The drawing under review shows one solid part. Ordinate dimensions are in mm from its lowest x, y, z. Coordinates: 2 decimals unless noted, no trailing zeros. Order: outer loops, then holes, each group sorted by start corner. A loop starts at its lowest first (then second) coordinate and runs counter-clockwise, first axis right, second up.
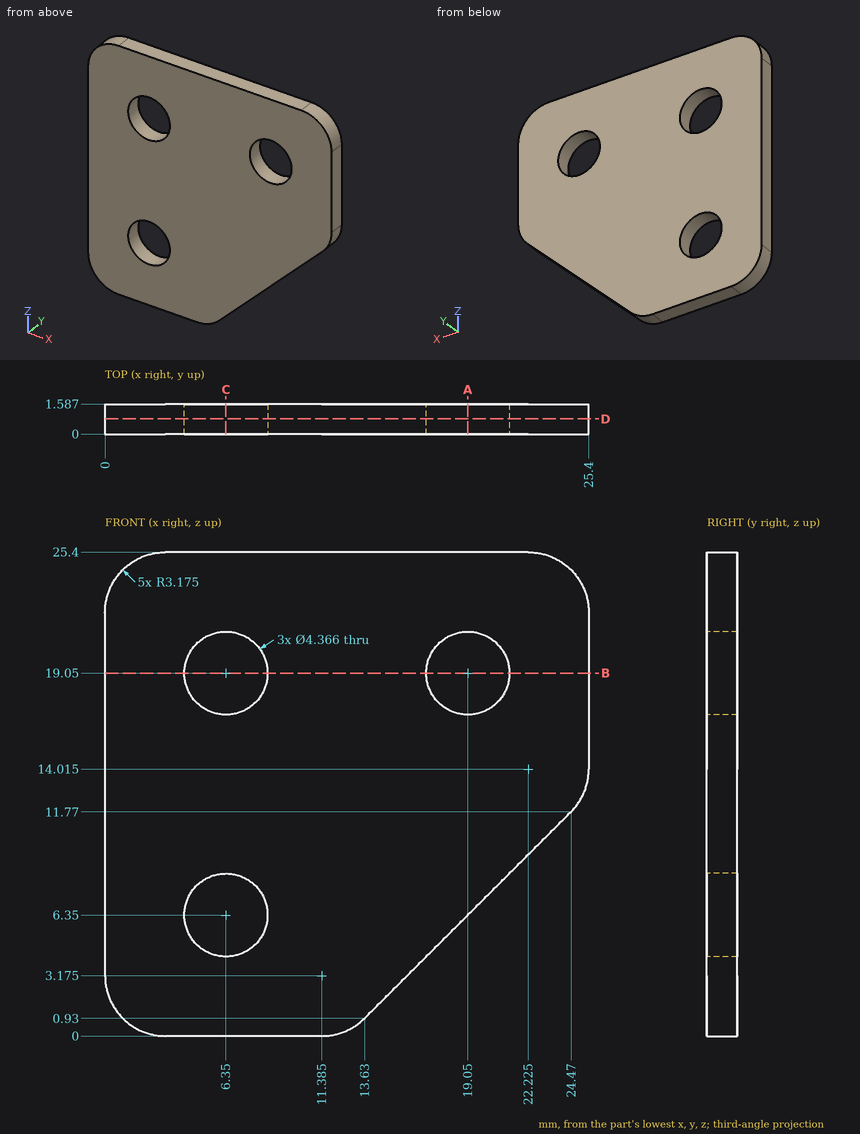
(1) Consider section B-B (z = 19.05). Give the boundary of the cut face in (x, y).
(2) Consider section D-D (y = 0.8). Give the number of separate pieces and of enclosed holes in the cut face, then the cut area to 3 significant figures.
(3) Insertion check: pin 1 Ø2.5 at (x, z) = (6.35, 19.05) entering from +Y. The pin has a flat end and moves straight along its axis. Give the tip position at first contact, or say it passes through.
(4) Consider section C-C (x = 6.35). Give the boundary of the cut face in (y, z).
(5) Wall thickness on line 1 (Z direction, x = 6.35, y = 0.9); line 2 (X direction, y = 0.9, z = 19.25); line 3 (X direction, y = 0.35, z = 20) (1 decimal): over which ranges is each line inside the solid? List them lowest first.
(6) Consider section A-A (x = 19.05). Give the boundary of the cut face in (y, z), then the cut area to 3 significant figures.
Findings:
1. outline: (0, 0) - (4.17, 0) - (4.17, 1.59) - (0, 1.59) - close; (8.53, 0) - (16.87, 0) - (16.87, 1.59) - (8.53, 1.59) - close; (21.23, 0) - (25.4, 0) - (25.4, 1.59) - (21.23, 1.59) - close
2. separate pieces: 1
2. enclosed holes: 3
2. area: 513 mm2
3. pin 1: passes through
4. outline: (0, 0) - (1.59, 0) - (1.59, 4.17) - (0, 4.17) - close; (0, 8.53) - (1.59, 8.53) - (1.59, 16.87) - (0, 16.87) - close; (0, 21.23) - (1.59, 21.23) - (1.59, 25.4) - (0, 25.4) - close
5. line 1: z = 0 to 4.17, 8.53 to 16.87, 21.23 to 25.4
5. line 2: x = 0 to 4.18, 8.52 to 16.88, 21.22 to 25.4
5. line 3: x = 0 to 4.4, 8.3 to 17.1, 21 to 25.4
6. outline: (0, 6.35) - (1.59, 6.35) - (1.59, 16.87) - (0, 16.87) - close; (0, 21.23) - (1.59, 21.23) - (1.59, 25.4) - (0, 25.4) - close
6. area: 23.3 mm2
